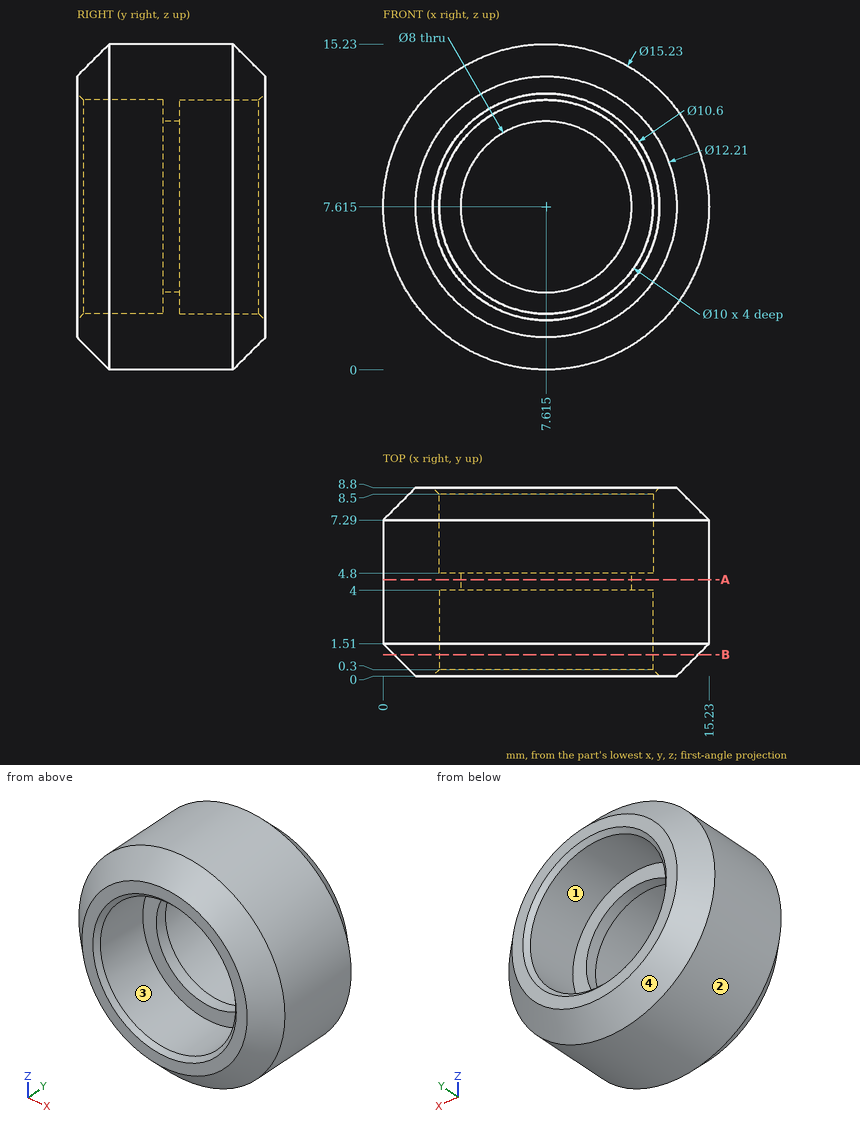
Study the drawing (mm; zero at the part's minimum x, y, z) and answer. A direction names the side the tool comes from. Round coordinates to 2 decimals unless told otherwise and drop trailing zeros. Loops run counter-clockwise (first coordinate to the right, second up) from the corner with the lowest first, then second, coordinate; pieces in that order, holes last.
Q1. Which of the six approach directions +Z, -Z, +X, -X, +Y, -Y give full straight-line access (tool end or side, diameter ignored) to the marked faces 3 and 4?
Q2. Find the intervals of material crossed by line 1 (X direction, y = 8.25, z = 7.75); line 2 (X direction, y = 7.5, z = 4); line 3 (Z direction, x = 12, y = 8.25), in increasing order.
Q3. For a pull along X with two mould halves and no side action, classify the marked faces 1 and 2 as released by +X, released by -X, zero draft, split by the parting line, or undercut.
Q4. Given pin 1 Ø5 at (x, y) = (12, 4) entering from +Z; pin 2 Ø2 at (x, z) = (11.5, 9) entering from +Y; pin 3 Ø8 at (x, z) = (7.5, 7) entering from -Y, each flat-ended and moving along its own axis, determine where each tip first touches the part or whether it passes through.
Q5. Section A-A, the plane y = 4.5 is taken. Determine the outline of the cut face in (x, z) (3 decimals), then the cut area to 3 significant figures.
Q6. Section B-B, the plane y = 1 is taken. Determine the outline of the cut face in (x, z) (3 decimals).
Completed:
1. face 3: -Y
1. face 4: +Y
2. line 1: x = 0.96 to 2.62, 12.61 to 14.27
2. line 2: x = 1.15 to 4.16, 11.07 to 14.08
2. line 3: z = 2.61 to 5.21, 10.02 to 12.62
3. face 1: undercut
3. face 2: split by the parting line
4. pin 1: stops at z = 14.99
4. pin 2: stops at y = 8.62
4. pin 3: stops at y = 4
5. outline: circle Ø15.23 at (7.615, 7.615); hole circle Ø8 at (7.615, 7.615)
5. area: 132 mm2
6. outline: circle Ø14.21 at (7.615, 7.615); hole circle Ø10 at (7.615, 7.615)
